Verification items for this drawing (mm, ordinates from the low corner). A direction names the side the tool comes from. Give positions to 0.01 mm unless a question says otherwise; leave off trailing zeros. Order: outer loops, then holes, each group sorted by start corner. A loop starts at its lowest first (then second) coordinate and runs counter-clockwise, first axis right, second up. Notation, with made-up numbers: (9, 59) -> (57, 59) arc R5 cw to (57, 68) -> close; hole circle Ø6 at (15, 84). An arc over 180 degrees is marked (long way). One line per question, with ' | ' between items.
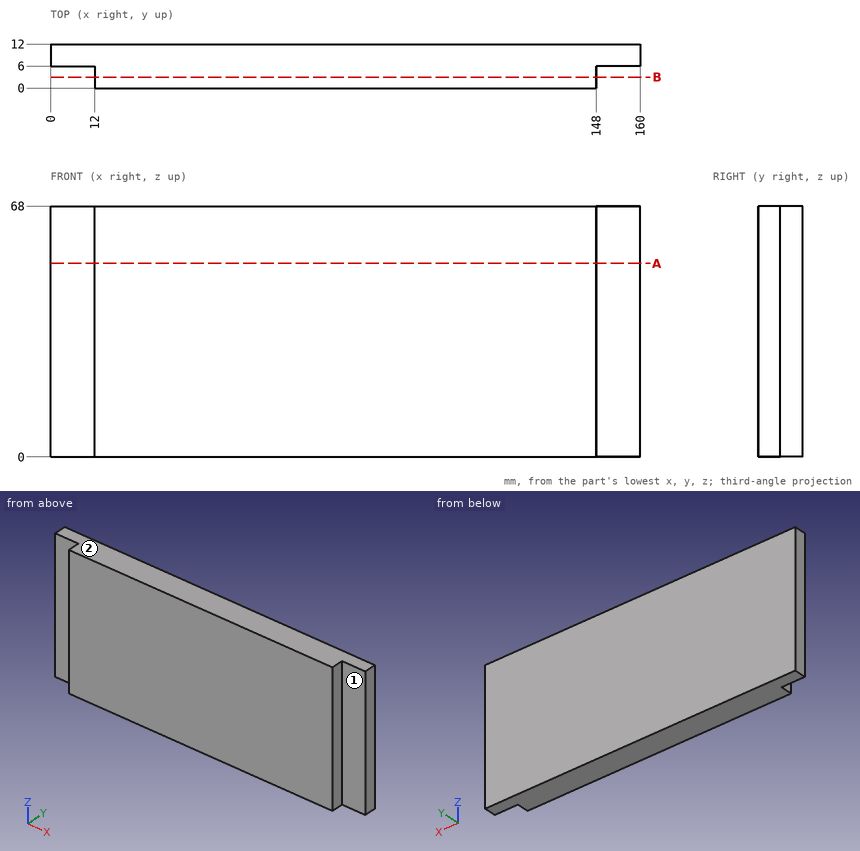
Q1. Access from +Z, -Z, +X, -X, +Y, -Y to the whole of each face (thin tool, end or side, straight path). Record for the marked faces 1 and 2.
Result sheet:
face 1: +Z, -Z, +X, -Y | face 2: +Z, +X, -X, +Y, -Y
Q2. Section check A-A (z = 52.5). Enter the section's corners in (x, y), and give its area (3 significant figures).
Result sheet:
outline: (0, 6) -> (12, 6) -> (12, 0) -> (148, 0) -> (148, 6) -> (160, 6) -> (160, 12) -> (0, 12) -> close | area: 1,780 mm2
Q3. Thickness scan on line 1 (X direction, y = 2, z = 50); line 2 (Y direction, x = 154.5, z = 32). Record the ranges inside material, lowest first.
Result sheet:
line 1: x = 12 to 148 | line 2: y = 6 to 12
Q4. Depth check by flat-ended pin: pin 1 Ø3.5 at (x, z) = (151.5, 26.5) entering from -Y; pin 2 Ø1.5 at (y, z) = (5, 51.5) entering from -X; pin 3 Ø1 at (x, y) = (109, 10) entering from -Z; pin 4 Ø3 at (y, z) = (3, 46) entering from +X. Enter the tip coordinate at first touch or a pass-through.
Result sheet:
pin 1: stops at y = 6 | pin 2: stops at x = 12 | pin 3: stops at z = 0 | pin 4: stops at x = 148
Q5. Section check B-B (y = 3). Enter the section's corners in (x, z), and give its area (3 significant figures).
Result sheet:
outline: (12, 0) -> (148, 0) -> (148, 68) -> (12, 68) -> close | area: 9,250 mm2
